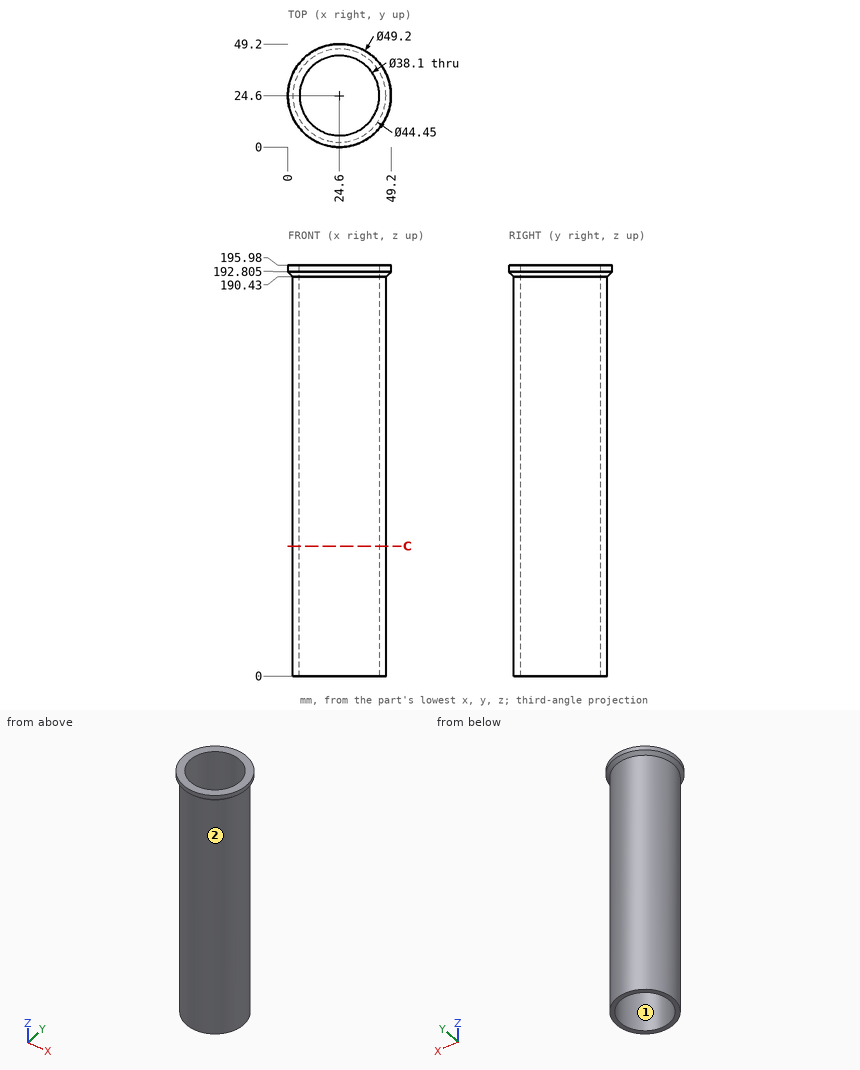
The figure shows three views and two pictorial views of one solid part (mm, origin at its lowest corner). Answer the questions. Give positions to 0.01 mm unless a question says otherwise; leave off trailing zeros. Loops run counter-clockwise (first coordinate to the right, second up) from the corner with the lowest first, then second, coordinate; pieces in that order, holes last. Notation, with made-up numbers: (37.5, 51.25) - (75.5, 51.25) arc R17 ccw to (75.5, 73.25) - close; hole circle Ø7 at (37, 12.25). An arc over 180 degrees is marked (long way). Answer in a Markdown table with one row per item.
(1) Consider L1, parallel to X at y = 24, z = 76; L2, parallel to Y at x = 24.6, z = 76.5 (3 decimals); L3, parallel to Y at x = 38, z = 124. Determine where each line is inside the solid, lowest interval first. Write a range as [from, to].
Results list:
| item | result |
|---|---|
| L1 | x = [2.38, 5.56], [43.64, 46.82] |
| L2 | y = [2.375, 5.55], [43.65, 46.825] |
| L3 | y = [6.87, 11.06], [38.14, 42.33] |
(2) Section C-C (z = 62) is taken. Give the vertices of the cut face in (x, y) (3 decimals).
Results list:
| item | result |
|---|---|
| outline | circle Ø44.45 at (24.6, 24.6); hole circle Ø38.1 at (24.6, 24.6) |
(3) Flat-ended cylindrical pins translate along their axes: pin 1 Ø4 at (x, z) = (39.5, 127) entering from +Y; pin 2 Ø1.5 at (y, z) = (30, 60.5) entering from +X; pin 3 Ø10 at (x, z) = (8.5, 136) entering from +Y (1 decimal). Find the tip coordinate at first contact, or state that the pin passes through.
Results list:
| item | result |
|---|---|
| pin 1 | stops at y = 42.7 |
| pin 2 | stops at x = 46.33 |
| pin 3 | stops at y = 43.9 |
(4) For a pull along X with two mould halves and no side action, classify the marked faces 1 and 2 as pulls with the +X half, pulls with the -X half, needs draft (parallel to the pull), parting line crosses it, or undercut.
Results list:
| item | result |
|---|---|
| face 1 | undercut |
| face 2 | parting line crosses it |
